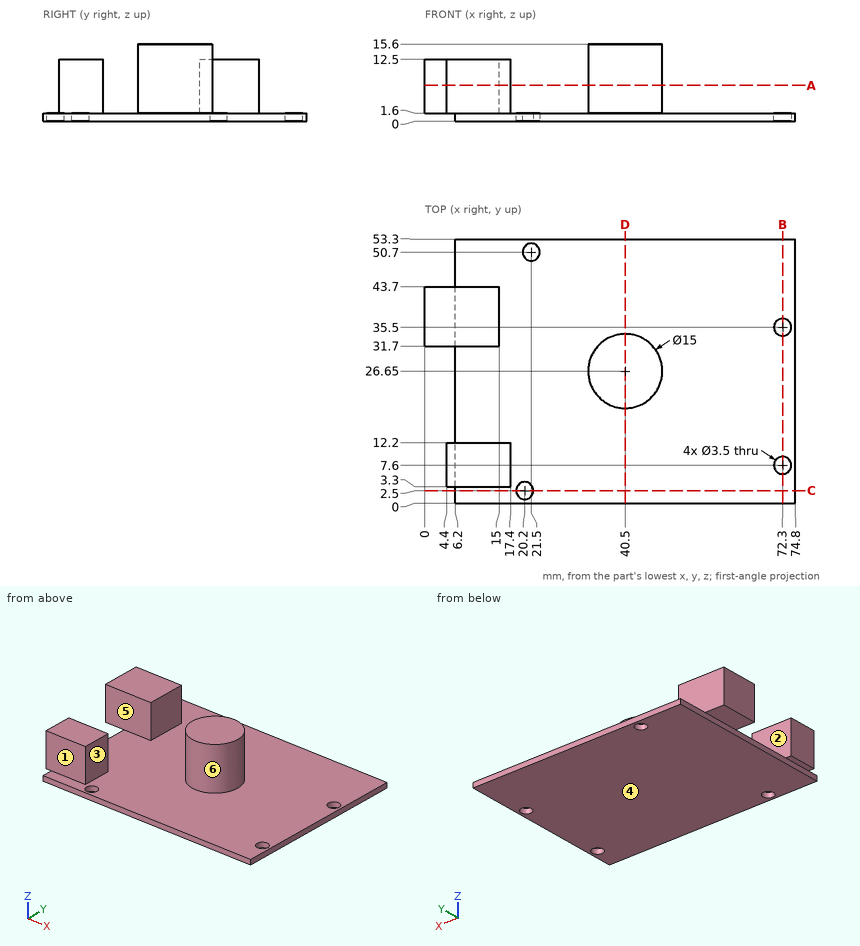
Geometry check sheet. Reference: drawing and pictorial views, mm from the part's lowest x, y, z. A direction names the side the tool comes from. Round coordinates to 2 decimals unless told otherwise and drop trailing zeros. Loops run counter-clockwise (first coordinate to the right, second up) from the corner with the lowest first, then second, coordinate; pieces in that order, holes last.
1. Mould release check, pull along Y, two halves, no side actions. Record for the marked faces 4, 5 and 6: released by +Y, released by -Y, zero draft, split by the parting line, or undercut.
2. Gauge pin test, flat ends, axial feed: pin 1 Ø1.8 at (y, z) = (24, 1) entering from -X; pin 2 Ø4.5 at (x, y) = (21.5, 50.7) entering from +Z; pin 3 Ø12 at (x, y) = (29.5, 12) entering from -Z; pin 4 Ø1.9 at (x, y) = (2, 37.5) entering from -Z. Record the tip position at first contact, or that the pin passes through.
3. Set-up check for the marked faces 1, 2 and 3: record each of +Z, -Z, +X, -X, +Y, -Y from which the full face is reachable in a straight line by a thin tool's end or side.
4. Sectioned sample at C-C on y = 2.5. Record the boundary of the cut face in (x, z), and give its area (3 significant figures).
5. Sectioned sample at D-D on x = 40.5. Record the boundary of the cut face in (y, z).
6. Sectioned sample at B-B on x = 72.3. Record the boundary of the cut face in (y, z).
7. Sectioned sample at A-A on z = 7.25. Record the boundary of the cut face in (x, y), and give its area (3 significant figures).
8. Scan lines: probe 1 along Y at (x, z) = (11, 11); probe 2 along Y at (x, z) = (20.2, 0.6); probe 3 along X at (y, z) = (50.7, 0.85). Record each from-to range of solid material in increasing order.
Recorded:
1. face 4: zero draft
1. face 5: undercut
1. face 6: split by the parting line
2. pin 1: stops at x = 6.2
2. pin 2: stops at z = 1.6
2. pin 3: stops at z = 0
2. pin 4: stops at z = 1.6
3. face 1: +Z, +X, -X, -Y
3. face 2: +Z, +X, -X
3. face 3: +Z, +X, +Y, -Y
4. outline: (6.2, 0) - (18.45, 0) - (18.45, 1.6) - (6.2, 1.6) - close; (21.95, 0) - (74.8, 0) - (74.8, 1.6) - (21.95, 1.6) - close
4. area: 104 mm2
5. outline: (0, 0) - (53.3, 0) - (53.3, 1.6) - (34.15, 1.6) - (34.15, 15.6) - (19.15, 15.6) - (19.15, 1.6) - (0, 1.6) - close
6. outline: (0, 0) - (5.85, 0) - (5.85, 1.6) - (0, 1.6) - close; (9.35, 0) - (33.75, 0) - (33.75, 1.6) - (9.35, 1.6) - close; (37.25, 0) - (53.3, 0) - (53.3, 1.6) - (37.25, 1.6) - close
7. outline: (0, 31.7) - (15, 31.7) - (15, 43.7) - (0, 43.7) - close; (4.4, 3.3) - (17.4, 3.3) - (17.4, 12.2) - (4.4, 12.2) - close; circle Ø15 at (40.5, 26.65)
7. area: 472 mm2
8. probe 1: y = 3.3 to 12.2, 31.7 to 43.7
8. probe 2: y = 0 to 0.75, 4.25 to 49.53, 51.87 to 53.3
8. probe 3: x = 6.2 to 19.75, 23.25 to 74.8
